from build123d import *

# Parameters (mm, degrees)
SKETCH1_W           = 40
SKETCH1_H           = 12.1
BOSS_EXTRUDE1_DEPTH = 3
SKETCH2_W           = 40
SKETCH2_H           = 7
SKETCH2_H_2         = 3
BOSS_EXTRUDE2_DEPTH = 10
SKETCH3_W           = 10.2
SKETCH3_H           = 3.2
CUT_EXTRUDE1_DEPTH  = 44.765397291
SKETCH5_W           = 4
SKETCH5_H           = 10
CUT_EXTRUDE3_DEPTH  = 25
SKETCH6_R           = 4.5
CUT_EXTRUDE4_DEPTH  = 3
FILLET3_R           = 10
FILLET1_R           = 0.4


with BuildPart() as part:
    # Sketch1 → Boss-Extrude1 (new body)
    with BuildSketch(Plane(origin=(0, 0, 0), x_dir=(1, 0, 0), z_dir=(0, 1, 0))):
        with Locations((20, -6.05)):
            Rectangle(SKETCH1_W, SKETCH1_H)
    extrude(amount=BOSS_EXTRUDE1_DEPTH)

    # Sketch2 → Boss-Extrude2 (add)
    with BuildSketch(Plane(origin=(0, 3, 0), x_dir=(1, 0, 0), z_dir=(0, 1, 0))):
        with Locations((20, -3.5)):
            Rectangle(SKETCH2_W, SKETCH2_H)
        with Locations((20, -10.6)):
            Rectangle(SKETCH2_W, SKETCH2_H_2)
    extrude(amount=BOSS_EXTRUDE2_DEPTH)

    # Sketch3 → Cut-Extrude1 (cut, through all)
    with BuildSketch(Plane(origin=(0, 0, 0), x_dir=(-1, 0, 0), z_dir=(0, 0, -1))):
        with Locations((-10, 3.6)):
            Rectangle(SKETCH3_W, SKETCH3_H)
    extrude(amount=-CUT_EXTRUDE1_DEPTH, mode=Mode.SUBTRACT)

    # Sketch5 → Cut-Extrude3 (cut)
    with BuildSketch(Plane.ZY):
        with Locations((5, 8)):
            Rectangle(SKETCH5_W, SKETCH5_H)
    extrude(amount=-CUT_EXTRUDE3_DEPTH, mode=Mode.SUBTRACT)

    # Sketch6 → Cut-Extrude4 (cut)
    with BuildSketch(Plane(origin=(0, 0, 0), x_dir=(-1, 0, 0), z_dir=(0, 0, -1))):
        with Locations((-14.588737144, 12.45970207)):
            Circle(SKETCH6_R)
    extrude(amount=-CUT_EXTRUDE4_DEPTH, mode=Mode.SUBTRACT)

    # Fillet3
    fillet3_edges = [part.edges().sort_by_distance(p)[0] for p in [
        (10.121290653, 13, 1.5),
    ]]
    fillet(fillet3_edges, radius=FILLET3_R)

    # Fillet1
    fillet1_edges = [part.edges().sort_by_distance(p)[0] for p in [
        (0, 3, 6.05),
        (40, 8, 7),
        (0, 13, 1.5),
        (40, 13, 3.5),
        (29.528091817, 13, 0),
        (40, 3, 8.05),
        (0, 8, 9.1),
        (40, 8, 9.1),
        (0, 13, 10.6),
        (20, 13, 12.1),
        (40, 13, 10.6),
        (20, 13, 9.1),
        (15.1, 3.6, 12.1),
        (10, 5.2, 12.1),
        (4.9, 3.6, 12.1),
        (10, 2, 12.1),
        (15.1, 3.6, 0),
        (10, 2, 0),
        (4.9, 3.6, 0),
        (20, 0, 0),
        (10, 5.2, 0),
        (40, 0, 6.05),
        (20, 0, 12.1),
        (0, 0, 6.05),
        (32.5, 13, 7),
        (32.5, 3, 7),
        (25, 8, 7),
        (25, 3, 5),
        (25, 8, 3),
        (25, 13, 5),
        (22.028091817, 13, 3),
        (0, 8, 3),
        (0, 6.5, 0),
        (40, 6.5, 0),
        (40, 6.5, 12.1),
        (0, 6.5, 12.1),
        (16.405345244, 8.342672193, 3),
        (19.056183635, 13, 1.5),
        (16.405345244, 8.342672193, 0),
        (1.79973399, 13, 3),
        (7.768441198, 12.089535869, 3),
        (1.79973399, 13, 0),
        (7.768441198, 12.089535869, 0),
    ]]
    fillet(fillet1_edges, radius=FILLET1_R)


solid = part.part
Input: part model. Units: mm. Frame: model coordinates. A direction names the side the tool comes from. Coordinates: 2 decimals unless noted, no trailing zeros. Write each loop counter-clockwise with the first axis right and the second up, starting at its lowest first coordinate (ties: lowest second). Pieces come first, ordered by that corner, then holes. Notation, with made-up numbers: M 74,89 L 124,89 A22 cw 124,97 Z; hole C 54.25,20 d10. An arc over 180 degrees is marked long. Answer as a JSON object with one key per item and string values. Group by question number.
(1) Ray query, line 1 along Z through (x, y) = (31.5, 6); line 2 along Z through (x, y) = (22, 6.5); line 3 along Z through (x, y) = (8.5, 12). Return the intervals inside material, ascending. Write a range as [from, to].
(2) Section B-B on z = 8. Output: boundary loops of the cut face in (x, y).
(3) Section C-C on x = 23. Output: boundary loops of the cut face in (y, z), plus the area to 3 significant figures.
(4) Set-up query: faces 4 (the face through (4.9, 2.5, 6)), 5 (the face through (20, 8, 9.1)), 6 (the face through (7.823, 12.064, 1.485)), 7 (the face through (40, 6, 6)), 8 (the face through (22, 3, 7)). Return all of +Z, -Z, +X, -X, +Y, -Y with unobstructed straight access to the full face (end or side cutting, diameter ignored); none if empty.
(5) Section A-A on y = 7. Output: boundary loops of the cut face in (x, z), plus the area to 3 significant figures.
(6) Section D-D on y = 4. Give the number of separate pieces and of enclosed holes in the cut face, plus the area to 3 significant figures.
(7) Mould query, pull axis Y, two halves, no side actions, for faces 1 (the face through (32, 8, 7)), 2 (the face through (10, 2, 6)), 3 (the face through (20, 13, 11)). Classes: pulls with the +Y half, pulls with the -Y half, needs draft (parallel to the pull), parting line crosses it, or undercut.
(8) Contact query for flat-ended pins moving along their axis: P1, Ø5, axis at x = 2, z = 6, coming from the +Y side; P2, Ø1.6, axis at y = 9.5, z = 6, coming from the -X side. Output: stop coordinate, or through.
Result set:
{
 "1": {"line 1": "z = [0, 7], [9.1, 12.1]", "line 2": "z = [0, 3], [9.1, 12.1]", "line 3": "z = [9.1, 12.1]"},
 "2": {"outline": "M 0,0.4 A0.4 ccw 0.4,0 L 39.6,0 A0.4 ccw 40,0.4 L 40,2.6 A0.4 ccw 39.6,3 L 15.1,3 L 15.1,2 L 4.9,2 L 4.9,3 L 0.4,3 A0.4 ccw 0,2.6 Z"},
 "3": {"outline": "M 0,0.4 A0.4 ccw 0.4,0 L 12.6,0 A0.4 ccw 13,0.4 L 13,2.6 A0.4 ccw 12.6,3 L 3,3 L 3,9.1 L 12.6,9.1 A0.4 ccw 13,9.5 L 13,11.7 A0.4 ccw 12.6,12.1 L 0.4,12.1 A0.4 ccw 0,11.7 Z", "area": "96.1 mm2"},
 "4": {"face 4": "+Z, -Z", "face 5": "+X, -X, +Y", "face 6": "-Z, +Y", "face 7": "+Z, -Z, +X, +Y, -Y", "face 8": "-X, +Y"},
 "5": {"outline": "M 0,0.4 A0.4 ccw 0.4,0 L 39.6,0 A0.4 ccw 40,0.4 L 40,6.6 A0.4 ccw 39.6,7 L 25.4,7 A0.4 ccw 25,6.6 L 25,3.4 A0.4 cw 24.6,3 L 0.4,3 A0.4 ccw 0,2.6 Z; M 0,9.5 A0.4 ccw 0.4,9.1 L 39.6,9.1 A0.4 ccw 40,9.5 L 40,11.7 A0.4 ccw 39.6,12.1 L 0.4,12.1 A0.4 ccw 0,11.7 Z", "area": "300 mm2"},
 "6": {"separate pieces": "4", "enclosed holes": "0", "area": "238 mm2"},
 "7": {"face 1": "needs draft", "face 2": "undercut", "face 3": "pulls with the +Y half"},
 "8": {"P1": "stops at y = 3", "P2": "stops at x = 25"}
}
